Verification items for this drawing (mm, ordinates from the low corner). A direction names the side the tool comes from. Coordinates: 2 decimals unless noted, no trailing zeros. Loops run counter-clockwise (first coordinate to the right, second up) from the corner with the lowest first, then second, coordinate; pieces in that order, holes last. Notation, with made-up numbers: M 54.25,33 L 75.25,33 A28 cw 75.25,65 Z; hole C 24.25,-16.5 d6. An arc over 180 degrees is marked long. Return JSON: item names as keys, results as strings.
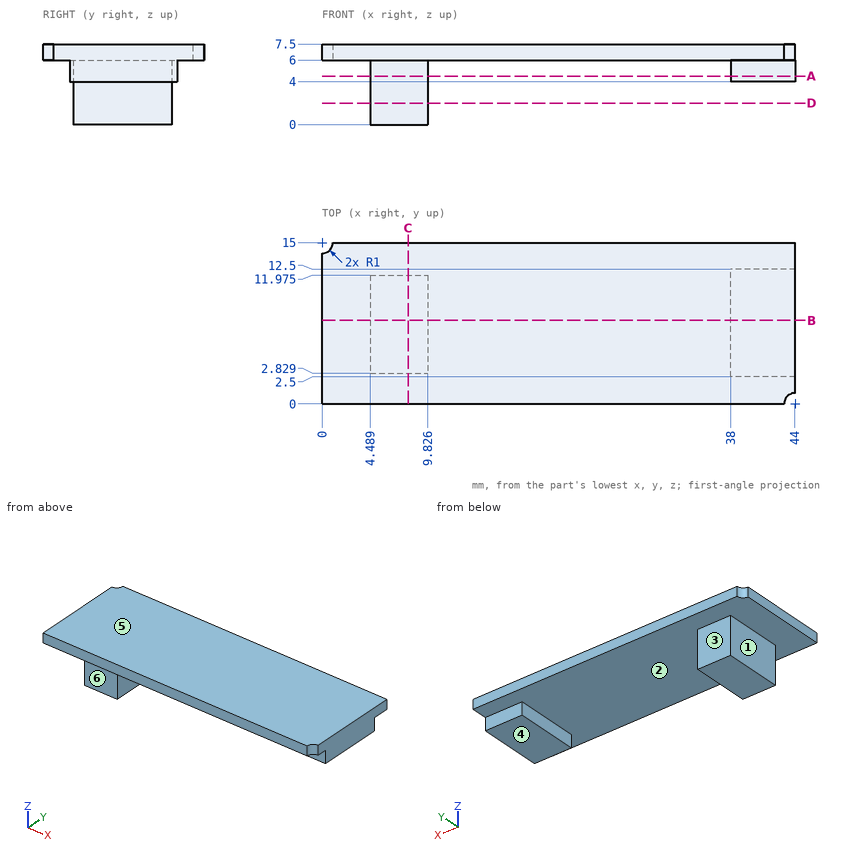
1) Section check C-C on x = 8. Record the cut outline in (y, z) (1 decimal).
Answers:
{"outline": "M 0,6 L 2.8,6 L 2.8,0 L 12,0 L 12,6 L 15,6 L 15,7.5 L 0,7.5 Z"}
2) Draft check along X on the marked faces 1, 2 and 3. Enter one of: +X half, -X half, draft (parallel to the pull), parting line (faces both ways), or undercut.
Answers:
{"face 1": "-X half", "face 2": "undercut", "face 3": "draft"}
3) Scan lines: line 1 along X through (y, z) = (5.75, 3); line 2 along X through (y, z) = (5.25, 5.5); line 3 along Z through (x, y) = (7.5, 1). Record each from-to range of solid material in increasing order. Write a range as [from, to].
Answers:
{"line 1": "[4.49, 9.83]", "line 2": "[4.49, 9.83], [38, 44]", "line 3": "[6, 7.5]"}
4) Set-up check for the marked faces 4, 5 and 6: record each of +Z, -Z, +X, -X, +Y, -Y from which the full face is reachable in a straight line by a thin tool's end or side.
Answers:
{"face 4": "-Z, +X, +Y, -Y", "face 5": "+Z, +X, -X, +Y, -Y", "face 6": "-Z, -X, -Y"}
5) Section check A-A on z = 4.5. Record the cut outline in (x, y) (1 decimal).
Answers:
{"outline": "M 4.5,2.8 L 9.8,2.8 L 9.8,12 L 4.5,12 Z; M 38,2.5 L 44,2.5 L 44,12.5 L 38,12.5 Z"}
6) Go/stop test with flat-tipped pins: pin 1 Ø0.6 at (y, z) = (5.5, 4.5) entering from -X; pin 2 Ø3 at (x, y) = (40.5, 8.5) entering from -Z; pin 3 Ø1.6 at (x, z) = (6, 4) entering from -Y. Record where each tip stops, or that it passes through.
Answers:
{"pin 1": "x = 4.49", "pin 2": "z = 4", "pin 3": "y = 2.83"}
7) Section check D-D on z = 2. Record the cut outline in (x, y) (1 decimal).
Answers:
{"outline": "M 4.5,2.8 L 9.8,2.8 L 9.8,12 L 4.5,12 Z"}
8) Section check B-B on y = 7.75. Record the cut outline in (x, z).
Answers:
{"outline": "M 0,6 L 4.49,6 L 4.49,0 L 9.83,0 L 9.83,6 L 38,6 L 38,4 L 44,4 L 44,7.5 L 0,7.5 Z"}
